Can you work these out from the model? Positions are in its coordinate system, mm. Face numbers are marked on the shaded views. A direction names the side the tool comes from. Round coordinates to 2 decimals unless told otherwise and drop trailing zeros. Order: outer loops, then holes, each group sorted by start corner. A loop starts at its lowest first (then second) coordinate and runs counter-clockwise, first axis right, second up. Notation, with made-up numbers: (54, 7.25) - (84, 7.25) arc R26 ccw to (84, 28.25) - close; hole circle Ø6 at (19, -31). An arc over 180 degrees is marked (long way). Write item = value, one per line.
from build123d import *

# Parameters (mm, degrees)
BOSS_EXTRUDE1_DEPTH = 650.24
FILLET1_R           = 25.4
BOSS_EXTRUDE2_DEPTH = 0.254
SKETCH4_W           = 599.44
SKETCH4_H           = 333.15660942
BOSS_EXTRUDE3_DEPTH = 0.00254
BOSS_EXTRUDE4_DEPTH = 86.36
SKETCH6_R           = 44.45
CUT_EXTRUDE1_DEPTH  = 99.568
SKETCH7_W           = 17.431192508
SKETCH7_H           = 33.637597394
SKETCH7_W_2         = 6.35
SKETCH7_H_2         = 27.707593027
SKETCH7_W_3         = 16.902871881
SKETCH7_W_4         = 15.731237492
SKETCH7_W_5         = 16.054307847
SKETCH7_R           = 1.896030158
CUT_EXTRUDE2_DEPTH  = 173.228


with BuildPart() as part:
    # Sketch1 → Boss-Extrude1 (new body)
    with BuildSketch(Plane.XY):
        with BuildLine():
            Line((0, 0), (25.4, 0))
            ThreePointArc((25.4, 0), (71.061606083, 228.6), (25.4, 457.2))
            Line((25.4, 457.2), (0, 457.2))
            Line((0, 457.2), (0, 0))
        make_face()
    extrude(amount=BOSS_EXTRUDE1_DEPTH)

    # Fillet1
    fillet1_edges = [part.edges().sort_by_distance(p)[0] for p in [
        (12.7, 457.2, 650.24),
        (12.7, 457.2, 0),
        (12.7, 0, 0),
        (12.7, 0, 650.24),
    ]]
    fillet(fillet1_edges, radius=FILLET1_R)

    # Sketch2 → Boss-Extrude2 (add)
    with BuildSketch(Plane.ZY):
        with BuildLine():
            Line((0, 69.440928173), (0, 25.4))
            ThreePointArc((0, 25.4), (7.439487758, 7.439487758), (25.4, 0))
            Line((25.4, 0), (624.84, 0))
            ThreePointArc((624.84, 0), (642.800512242, 7.439487758), (650.24, 25.4))
            Line((650.24, 25.4), (650.24, 69.440928173))
            Line((650.24, 69.440928173), (0, 69.440928173))
        make_face()
    extrude(amount=BOSS_EXTRUDE2_DEPTH)

    # Sketch4 → Boss-Extrude3 (add)
    with BuildSketch(Plane.ZY):
        with Locations((325.12, 265.22169529)):
            Rectangle(SKETCH4_W, SKETCH4_H)
    extrude(amount=BOSS_EXTRUDE3_DEPTH)

    # Sketch5 → Boss-Extrude4 (add, symmetric)
    with BuildSketch(Plane.XY.offset(325.12)):
        with BuildLine():
            Line((170.767248261, -51.198725882), (90.734414709, 202.070998511))
            ThreePointArc((90.734414709, 202.070998511), (82.810722474, 219.680826846), (71.027410341, 234.979340102))
            ThreePointArc((71.027410341, 234.979340102), (70.962867279, 239.439815668), (70.86488784, 243.899682046))
            ThreePointArc((70.86488784, 243.899682046), (86.537300589, 225.702245278), (96.789301226, 203.984333103))
            Line((96.789301226, 203.984333103), (176.83835346, -49.336716487))
            ThreePointArc((176.83835346, -49.336716487), (172.803446222, -72.154097904), (152.095027867, -82.55))
            Line((152.095027867, -82.55), (-25.704972133, -82.55))
            Line((-25.704972133, -82.55), (-25.704972133, -76.2))
            Line((-25.704972133, -76.2), (152.095027867, -76.2))
            ThreePointArc((152.095027867, -76.2), (167.697235419, -68.379202467), (170.767248261, -51.198725882))
        make_face()
    extrude(amount=BOSS_EXTRUDE4_DEPTH, both=True)

    # Sketch6 → Cut-Extrude1 (cut)
    with BuildSketch(Plane(origin=(200.66, 0, 0), x_dir=(0, 0, -1), z_dir=(1, 0, 0))):
        with Locations(Location((-327.103881197, 87.189356475, 0), (0, 0, 270))):
            Circle(SKETCH6_R)
    extrude(amount=-CUT_EXTRUDE1_DEPTH, mode=Mode.SUBTRACT)

    # Sketch7 → Cut-Extrude2 (cut)
    # profile 1 of 6: a face of its own
    with BuildSketch(Plane(origin=(200.66, 0, 0), x_dir=(0, 0, -1), z_dir=(1, 0, 0))):
        with Locations((-447.612414344, 67.453463266)):
            Rectangle(SKETCH7_W, SKETCH7_H)
        with Locations((-450.987768144, 67.846432455)):
            Rectangle(SKETCH7_W_2, SKETCH7_H_2, mode=Mode.SUBTRACT)
    # profile 2 of 6: a face of its own
    with BuildSketch(Plane(origin=(200.66, 0, 0), x_dir=(0, 0, -1), z_dir=(1, 0, 0))):
        with Locations((-425.36538215, 67.453463266)):
            Rectangle(SKETCH7_W_3, SKETCH7_H)
        with Locations((-428.061900395, 67.846432455)):
            Rectangle(SKETCH7_W_2, SKETCH7_H_2, mode=Mode.SUBTRACT)
    # profile 3 of 6: a face of its own
    with BuildSketch(Plane(origin=(200.66, 0, 0), x_dir=(0, 0, -1), z_dir=(1, 0, 0))):
        with Locations((-469.273629344, 67.453463266)):
            Rectangle(SKETCH7_W_4, SKETCH7_H)
        with Locations((-471.274687087, 67.846432455)):
            Rectangle(SKETCH7_W_2, SKETCH7_H_2, mode=Mode.SUBTRACT)
    # profile 4 of 6: a face of its own
    with BuildSketch(Plane(origin=(200.66, 0, 0), x_dir=(0, 0, -1), z_dir=(1, 0, 0))):
        with Locations((-490.246402014, 67.453463266)):
            Rectangle(SKETCH7_W_5, SKETCH7_H)
        with Locations((-492.809474486, 67.846432455)):
            Rectangle(SKETCH7_W_2, SKETCH7_H_2, mode=Mode.SUBTRACT)
    # profile 5 of 6: a face of its own
    with BuildSketch(Plane(origin=(200.66, 0, 0), x_dir=(0, 0, -1), z_dir=(1, 0, 0))):
        with BuildLine():
            Line((-506.422738648, 66.642270475), (-537.274582932, 66.642270475))
            ThreePointArc((-537.274582932, 66.642270475), (-538.544582932, 65.372270475), (-537.274582932, 64.102270475))
            Line((-537.274582932, 64.102270475), (-506.422738648, 64.102270475))
            ThreePointArc((-506.422738648, 64.102270475), (-505.152738648, 65.372270475), (-506.422738648, 66.642270475))
        make_face()
    # profile 6 of 6: a face of its own
    with BuildSketch(Plane(origin=(200.66, 0, 0), x_dir=(0, 0, -1), z_dir=(1, 0, 0))):
        with Locations((-547.498439967, 65.372270475)):
            Circle(SKETCH7_R)
    extrude(amount=-CUT_EXTRUDE2_DEPTH, mode=Mode.SUBTRACT)


solid = part.part
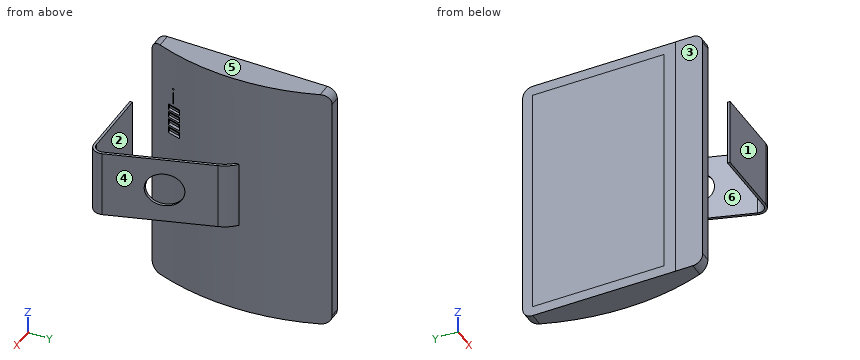
(1) Will these pins go through, and if not, where does the flat tip stop? P1, Ø2, axis at y = 374.5, z = 541, coming from the +X side; P2, Ø5, axis at y = 361.5, z = 504.5, coming from the +X side; P3, Ø6, axis at y = 65.37, z = 547.5, coming from the -X side.
Computed:
P1 = 53.15
P2 = 56.6
P3 = -0.25
(2) On a 3-axis mill with a long thin cutter (end or side, diameter ignored), from which of +Z, -Z, +X, -X, +Y, -Y can I reach the whole of each face in a straight line? I mean the marked faces 1, 2 and 3. Say none if no direction works.
Computed:
face_1 = +Z, -Z, +X, -X, -Y
face_2 = +Z, -Z, -X
face_3 = +Z, -Z, -X, +Y
(3) If I drill on line 1 (Y direction, x = 84, z = 245.5); line 2 (Y direction, x = 11.5, z = 147.5); line 3 (X direction, y = 175, z = 383), over which ranges is the centre line in solid material (lowest first)? Write a range as from..to.
Computed:
line_1 = -82.55..-76.2, 217.63..229.4
line_2 = 0..457.2
line_3 = 0..68.64, 99.29..105.95
(4) Thinking about a two-plate mould opening in X: for the marked faces 4, 5 and 6, which applies, +X half, -X half, draft (parallel to the pull), parting line (faces both ways), or undercut?
Computed:
face_4 = +X half
face_5 = draft
face_6 = undercut
(5) If we section it at A-A (x = 8.5): Write out the boundary of the cut face in (y, z).
Computed:
outline = (-82.55, 238.76) - (-76.2, 238.76) - (-76.2, 411.48) - (-82.55, 411.48) - close; (0, 25.4) arc R25.4 ccw to (25.4, 0) - (431.8, 0) arc R25.4 ccw to (457.2, 25.4) - (457.2, 624.84) arc R25.4 ccw to (431.8, 650.24) - (25.4, 650.24) arc R25.4 ccw to (0, 624.84) - close
(6) If we section it at C-C (x = 124): Write out the boundary of the cut face in (y, z).
Computed:
outline = (-82.55, 238.76) - (-76.2, 238.76) - (-76.2, 411.48) - (-82.55, 411.48) - close; (96.8, 238.76) - (117.87, 238.76) - (117.87, 294.94) arc R44.45 cw to (96.8, 283.71) - close; (96.8, 370.5) arc R44.45 cw to (117.87, 359.26) - (117.87, 411.48) - (96.8, 411.48) - close
